The model under review builds one solid part; all positions refer to its coordinate system, in mm. A direction names the side the tool comes from. Round coordinates to 2 decimals unless told otherwise and drop trailing zeros. Order: outer loops, then holes, each group sorted by start corner. A loop starts at its lowest first (then second) coordinate and runs counter-clockwise, first axis right, second up. Notation, with made-up numbers: M 83.5,38 L 130.5,38 A29 cw 130.5,74 Z; hole C 69.25,-3.75 d4. An arc over 180 degrees is marked long. Answer as a JSON object with one key per item and string values. Group by question number.
1. Mouldability with a two-part tool opening along Y and no side actions: class faces 1 (the face through (0, 0, 1.5)), 2 (the face through (0, 8.75, 4)), 3 (the face through (0, -8.75, 4)), 4 (the face through (35, 0, 4)) as released by +Y, released by -Y, zero draft, split by the parting line, or undercut.
2. Add section B-B on y = 0. State the section outline as (x, z) points.
3. To check wall thickness, follow probe 1 along X at (y, z) = (-2.5, 2); probe 2 along Y at (x, z) = (8, 7.25); probe 3 along X at (y, z) = (-6.75, 9.75). State the ranges of each line that lie inside material, in increasing order. Write a range as [from, to].
4. Machinability: for faces 5 (the face through (-32.106, 5.816, 4.458)), 6 (the face through (-34.24, -0.07, 4.25)), which of the approach directions +Z, -Z, +X, -X, +Y, -Y give a long, thin tool a straight path to every point of the face, cutting with its end or side? Answer none if there is none.
5. Add section A-A on z = 9.5. State the section outline as (x, y) points, and give its area (3 significant figures).
6. Clearance check with flat-ended pins moving along their axes: P1, Ø1.6, axis at x = -5.5, y = -5.5, coming from the +Z side; P2, Ø10, axis at x = 6, y = -6, coming from the +Z side. State where each tip first meets the part, or that it passes through.
7. Add section C-C on x = 2. State the section outline as (y, z) points, and give its area (4 significant figures).
```python
from build123d import *

# Parameters (mm, degrees)
F0_W     = 70
F0_H     = 17.5
F1_DEPTH = 7.5
F2_T     = -1.5
F4_DEPTH = 6
F6_DEPTH = 2.9
F7_R     = 3.25
F8_DEPTH = 70.001


with BuildPart() as f1:
    # F0 (on Top) → F1 (new body)
    with BuildSketch(Plane.XY):
        Rectangle(F0_W, F0_H)
    extrude(amount=F1_DEPTH)

    # F2
    f2_openings = [f1.faces().sort_by_distance(p)[0] for p in [
        (0, 0, 7.5),
    ]]
    offset(amount=F2_T, openings=f2_openings)

    # F3 (on face) → F4 (join, through all)
    with BuildSketch(Plane.XY.offset(1.5)):
        Polygon((-33.5, 7.25), (-33.5, 4.421573), (-30.671573, 7.25), align=None)
        Polygon((30.671573, 7.25), (33.5, 4.421573), (33.5, 7.25), align=None)
        Polygon((33.5, -7.25), (33.5, -4.421573), (30.671573, -7.25), align=None)
        Polygon((-33.5, -4.421573), (-33.5, -7.25), (-30.671573, -7.25), align=None)
    extrude(amount=F4_DEPTH)

    # F5 (on face) → F6 (join)
    with BuildSketch(Plane.XY.offset(7.5)):
        with BuildLine():
            ThreePointArc((-32.651472, 6.401472), (-32.499731, 6.628568), (-32.446447, 6.896447))
            ThreePointArc((-32.446447, 6.896447), (-33.793162, 7.164325), (-32.651472, 6.401472))
        make_face()
        with BuildLine():
            ThreePointArc((-32.651472, -6.401472), (-33.793162, -7.164325), (-32.446447, -6.896447))
            ThreePointArc((-32.446447, -6.896447), (-32.499731, -6.628568), (-32.651472, -6.401472))
        make_face()
        with BuildLine():
            ThreePointArc((32.651472, 6.401472), (33.414325, 6.249731), (33.846447, 6.896447))
            ThreePointArc((33.846447, 6.896447), (32.878568, 7.543162), (32.651472, 6.401472))
        make_face()
        with BuildLine():
            ThreePointArc((32.651472, -6.401472), (32.878568, -7.543162), (33.846447, -6.896447))
            ThreePointArc((33.846447, -6.896447), (33.414325, -6.249731), (32.651472, -6.401472))
        make_face()
    extrude(amount=F6_DEPTH)

    # F7 (on face) → F8 (cut, through all)
    with BuildSketch(Plane.YZ.offset(35)):
        with Locations((0, 7.5)):
            Circle(F7_R)
    extrude(amount=-F8_DEPTH, mode=Mode.SUBTRACT)


solid = f1.part
```
Recorded:
{
 "1": {"face 1": "undercut", "face 2": "released by +Y", "face 3": "released by -Y", "face 4": "zero draft"},
 "2": {"outline": "M -35,0 L 35,0 L 35,4.25 L 33.5,4.25 L 33.5,1.5 L -33.5,1.5 L -33.5,4.25 L -35,4.25 Z"},
 "3": {"probe 1": "x = [-35, -33.5], [33.5, 35]", "probe 2": "y = [-8.75, -7.25], [7.25, 8.75]", "probe 3": "x = [-33.83, -32.46], [32.46, 33.83]"},
 "4": {"face 5": "+Z", "face 6": "+Z, +X, -X"},
 "5": {"outline": "M -32.65,-6.4 A0.7 ccw long -32.45,-6.9 A0.7 ccw Z; M -32.65,6.4 A0.7 ccw -32.45,6.9 A0.7 ccw long Z; C 33.15,-6.9 d1.4; C 33.15,6.9 d1.4", "area": "6.16 mm²"},
 "6": {"P1": "stops at z = 1.5", "P2": "stops at z = 7.5"},
 "7": {"outline": "M -8.75,0 L 8.75,0 L 8.75,7.5 L 7.25,7.5 L 7.25,1.5 L -7.25,1.5 L -7.25,7.5 L -8.75,7.5 Z", "area": "44.25 mm²"}
}
